Can you work these out from the drawing? Everything is in mm from the part's minimum corner. A direction names the side the tool comes from. Round coordinates to 2 decimals unless told otherwise and drop trailing zeros. Write each loop counter-clockwise with the first axis right and the second up, starting at its lowest first coordinate (ties: lowest second). Pieces come first, ordered by that corner, then holes. Notation, with made-up numbers: M -9,16.25 L 12,16.25 A8 cw 12,28.25 Z; hole C 70.5,-27.75 d8. An arc over 180 degrees is marked long. Use one line per item in the form item = value. Start each with the question number.
Q1. I need wall thicknesses on line 1 along Z through (x, y) = (6.75, 2); line 2 along Z through (x, y) = (5.75, 0.5); line 3 along Y through (x, z) = (5.5, 30.25). Which ranges of each line are inside material? Lowest first, please. Write a range as from..to.
Q2. I want a section at A-A on y = 5.5. List the corners of the cut face in (x, z) for me, and give its area (3 significant figures).
Q3. I'm going to push flat-ended pins straight in: pin 1 Ø2 at (x, z) = (4, 18.5) entering from +Y; pin 2 Ø3.5 at (x, y) = (5.5, 5.5) entering from +Z; pin 3 Ø5 at (y, z) = (6.5, 5.5) entering from -X; pin 4 Ø1 at (y, z) = (5, 15) entering from +X. Where does each tip first touch, or does it pass through?
Q4. I want a section at B-B on x = 7. List the corners of the cut face in (y, z) for me, and give its area (3 significant figures).
Q5. I want a section at C-C on y = 2.25. List the corners of the cut face in (x, z) for me.
Q6. For the marked faces 5, 6 and 7, which set-ups out of +Z, -Z, +X, -X, +Y, -Y let a thin tool reach every point of the face, with its end or its side?
Q7. I want a section at D-D on z = 8. List the corners of the cut face in (x, y) for me, and give its area (4 significant figures).
Q8. We'd pull the mould along Z, two halves only. Please class the marked faces 1, 2, 3 and 4: +Z half, -Z half, draft (parallel to the pull), parting line (faces both ways), or undercut.
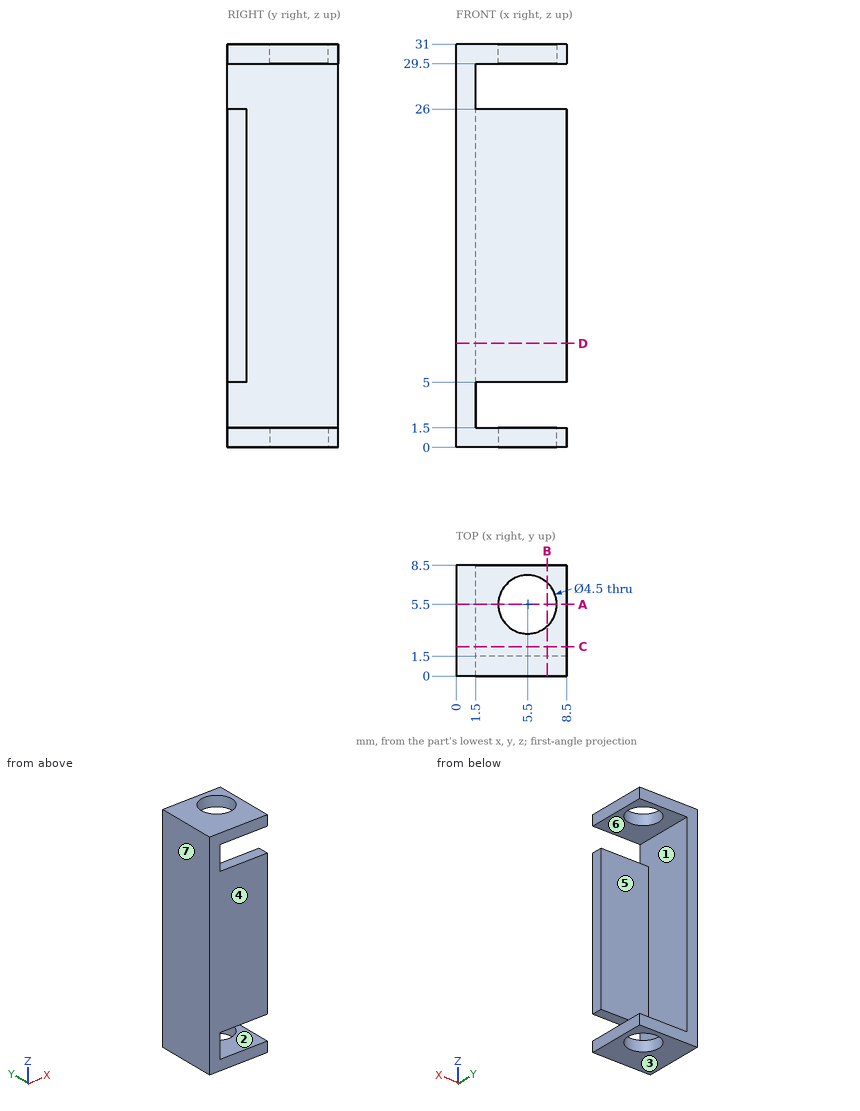
Reported:
q1.line_1 = 0..1.5, 29.5..31
q1.line_2 = 0..1.5, 5..26, 29.5..31
q1.line_3 = 0..3.25, 7.75..8.5
q2.outline = M 0,0 L 3.25,0 L 3.25,1.5 L 1.5,1.5 L 1.5,29.5 L 3.25,29.5 L 3.25,31 L 0,31 Z; M 7.75,0 L 8.5,0 L 8.5,1.5 L 7.75,1.5 Z; M 7.75,29.5 L 8.5,29.5 L 8.5,31 L 7.75,31 Z
q2.area = 54.0 mm^2
q3.pin_1 = 1.5
q3.pin_2 = through
q3.pin_3 = 0
q3.pin_4 = 1.5
q4.outline = M 0,0 L 3.82,0 L 3.82,1.5 L 0,1.5 Z; M 0,5 L 1.5,5 L 1.5,26 L 0,26 Z; M 0,29.5 L 3.82,29.5 L 3.82,31 L 0,31 Z; M 7.18,0 L 8.5,0 L 8.5,1.5 L 7.18,1.5 Z; M 7.18,29.5 L 8.5,29.5 L 8.5,31 L 7.18,31 Z
q4.area = 46.9 mm^2
q5.outline = M 0,0 L 8.5,0 L 8.5,1.5 L 1.5,1.5 L 1.5,29.5 L 8.5,29.5 L 8.5,31 L 0,31 Z
q6.face_5 = +X, +Y
q6.face_6 = +X, +Y, -Y
q6.face_7 = +Z, -Z, -X, +Y, -Y
q7.outline = M 0,0 L 8.5,0 L 8.5,1.5 L 1.5,1.5 L 1.5,8.5 L 0,8.5 Z
q7.area = 23.25 mm^2
q8.face_1 = undercut
q8.face_2 = undercut
q8.face_3 = -Z half
q8.face_4 = draft
